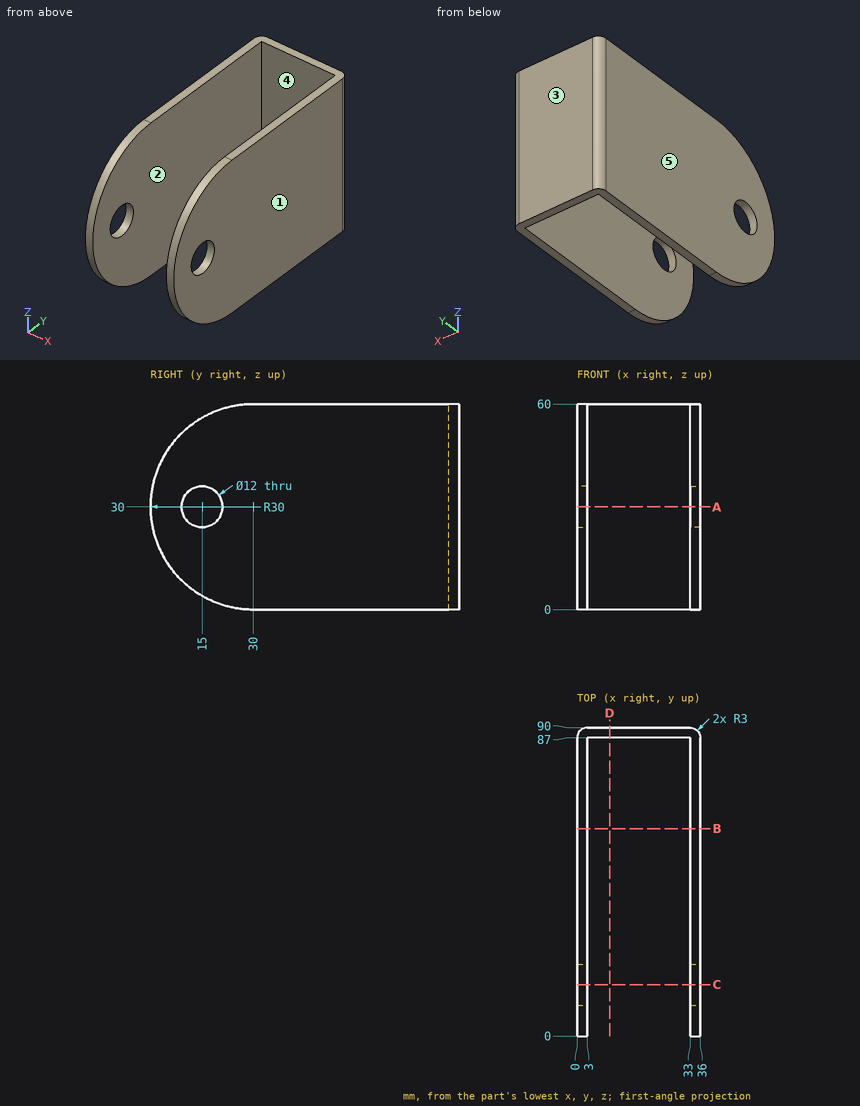
Answer from the drawing. Dimensions are ordinates in mm from the lowest x, y and z of the part. A direction names the side the tool comes from. Give positions to 0.01 mm unless a question says otherwise; leave off trailing zeros. Write each loop counter-clockwise with the first axis right and the second up, starting at its lowest first coordinate (ties: lowest second). Pieces come first, ordered by that corner, then holes.
1) For a pull along X with two mould halves and no side action, classify the marked faces 1, 2 and 3 as pulls with the +X half, pulls with the -X half, needs draft (parallel to the pull), parting line crosses it, or undercut.
2) Given P1, Ø14, axis at y = 15, z = 30, coming from the -X side; P2, Ø5, axis at x = 24.5, z = 41.5, coming from the -Y side; P3, Ø12, axis at x = 24, y = 63.5, coming from the +Z side, each flat-ended and moving along its own axis, determine where each tip first touches the part or whether it passes through.
3) A tool of negligible diameter and unlimited length cuts with its end or side. For the marked faces 4 and 5, from which of +Z, -Z, +X, -X, +Y, -Y can it reach the whole face along a straight path? Write none if from no direction.
4) Section C-C (y = 15) is taken. Write down the section's boundary in (x, z), and give its area (3 significant figures).
5) Find the intervals of material crossed by L1, parallel to X at y = 37, z = 15.5; L2, parallel to Y at x = 20, z = 56.5; L3, parallel to Y at x = 34, z = 30, in increasing order.
6) Section B-B (y = 60.5) is taken. Write down the section's boundary in (x, z).
7) Section A-A (z = 30) is taken. Write down the section's boundary in (x, y), and give its area (3 significant figures).
8) Section D-D (x = 9.5) is taken. Write down the section's boundary in (y, z), and give its area (3 significant figures).
Response:
1. face 1: pulls with the +X half
1. face 2: undercut
1. face 3: needs draft
2. P1: stops at x = 0
2. P2: stops at y = 87
2. P3: passes through
3. face 4: +Z, -Z, -Y
3. face 5: +Z, -Z, -X, +Y, -Y
4. outline: (0, 4.02) - (3, 4.02) - (3, 24) - (0, 24) - close; (0, 36) - (3, 36) - (3, 55.98) - (0, 55.98) - close; (33, 4.02) - (36, 4.02) - (36, 24) - (33, 24) - close; (33, 36) - (36, 36) - (36, 55.98) - (33, 55.98) - close
4. area: 240 mm2
5. L1: x = 0 to 3, 33 to 36
5. L2: y = 87 to 90
5. L3: y = 0 to 9, 21 to 89.83
6. outline: (0, 0) - (3, 0) - (3, 60) - (0, 60) - close; (33, 0) - (36, 0) - (36, 60) - (33, 60) - close
7. outline: (0, 0) - (3, 0) - (3, 9) - (0, 9) - close; (0, 21) - (3, 21) - (3, 87) - (33, 87) - (33, 21) - (36, 21) - (36, 87) arc R3 ccw to (33, 90) - (3, 90) arc R3 ccw to (0, 87) - close; (33, 0) - (36, 0) - (36, 9) - (33, 9) - close
7. area: 554 mm2
8. outline: (87, 0) - (90, 0) - (90, 60) - (87, 60) - close
8. area: 180 mm2
